from build123d import *

# Parameters (mm, degrees)
F0_W     = 12.7
F0_H     = 5.08
F1_DEPTH = 7.62
F2_R     = 2.53999


# Not quite as in the source:
# - a fillet or chamfer is up to 0.001 mm smaller than in the source, because OpenCascade refuses the exact size


with BuildPart() as f1:
    # F0 (on Top) → F1 (new body)
    with BuildSketch(Plane.XY):
        Polygon((-30.1547096223, 19.9307221919), (-30.1547096223, 5.9384261601), (-19.9947096223, 5.9384261601), (-19.9947096223, 14.8507221919), (-19.9947096223, 19.9307221919), align=None)
        Polygon((-19.9947096223, 5.9384261601), (-30.1547096223, 5.9384261601), (-30.1547096223, -6.7615738399), (33.3452903777, -6.7615738399), (33.3452903777, 5.9384261601), (23.1852903777, 5.9384261601), align=None)
        Polygon((23.1852903777, 14.8507221919), (23.1852903777, 5.9384261601), (33.3452903777, 5.9384261601), (33.3452903777, 19.9307221919), (23.1852903777, 19.9307221919), align=None)
        with Locations((-13.6447096223, 17.3907221919)):
            Rectangle(F0_W, F0_H)
        with Locations((16.8352903777, 17.3907221919)):
            Rectangle(F0_W, F0_H)
    extrude(amount=F1_DEPTH)

    # F2 (radius 2.54 in the source; OpenCascade refuses exactly that, so slightly less here)
    f2_edges = [f1.edges().sort_by_distance(p)[0] for p in [
        (1.59529, -6.761574, 7.62),
        (1.59529, 5.938426, 7.62),
        (-30.15471, 6.584574, 7.62),
        (33.34529, 6.584574, 7.62),
        (21.91529, 19.930722, 7.62),
        (-18.72471, 19.930722, 7.62),
        (21.91529, 19.930722, 0),
        (23.18529, 10.394574, 7.62),
        (16.83529, 14.850722, 7.62),
        (-13.64471, 14.850722, 7.62),
        (1.59529, -6.761574, 0),
        (-30.15471, 6.584574, 0),
        (33.34529, 6.584574, 0),
        (10.48529, 14.850722, 3.81),
        (10.48529, 19.930722, 3.81),
        (-7.29471, 14.850722, 3.81),
        (-7.29471, 19.930722, 3.81),
        (-19.99471, 10.394574, 7.62),
        (1.59529, 5.938426, 0),
        (-19.99471, 10.394574, 0),
        (16.83529, 14.850722, 0),
        (23.18529, 10.394574, 0),
        (-13.64471, 14.850722, 0),
        (10.48529, 17.390722, 0),
        (-7.29471, 17.390722, 0),
        (-18.72471, 19.930722, 0),
        (10.48529, 17.390722, 7.62),
        (-7.29471, 17.390722, 7.62),
    ]]
    fillet(f2_edges, radius=F2_R)


solid = f1.part
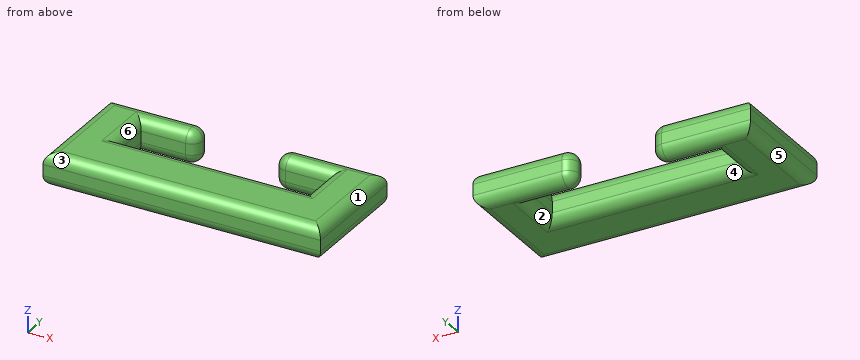
Check sheet for the modelled part. Datum: model origin and axes. Units: mm. Face numbers are marked on the shaded views. A direction names the side the tool comes from. Round coordinates to 2 decimals unless told otherwise and drop trailing zeros. Loops run counter-clockwise (first coordinate to the right, second up) from the corner with the lowest first, then second, coordinate; pieces in that order, holes last.
1. Gauge pin test, flat ends, axial feed: pin 1 Ø5 at (x, y) = (-17, 7.5) entering from -Z; pin 2 Ø3 at (x, y) = (-7, 5) entering from -Z; pin 3 Ø3 at (y, z) = (-4, 2) entering from +X; pin 4 Ø1.3 at (x, z) = (-4.5, 3.5) entering from +Y. Record the tip position at first contact, or that the pin passes through.
2. Scan lines: probe 1 along Y at (x, z) = (19, 3.5); probe 2 along X at (y, z) = (12, 4); probe 3 along X at (y, z) = (6.25, 5.25). Record each from-to range of solid material in increasing order.
3. Mould release check, pull along X, two halves, no side actions. Record for the marked faces 1, 2 and 3: released by +X, released by -X, zero draft, split by the parting line, or undercut.
4. Set-up check for the marked faces 4, 5 and 6: record each of +Z, -Z, +X, -X, +Y, -Y from which the full face is reachable in a straight line by a thin tool's end or side.
5. Sectioned sample at A-A on y = 10.5. Record the boundary of the cut face in (x, z), and give its area (3 significant figures).
6. Sectioned sample at D-D on x = -25. Record the boundary of the cut face in (y, z), and give its area (3 significant figures).
Recorded:
1. pin 1: stops at z = 0.57
1. pin 2: stops at z = 0
1. pin 3: stops at x = 33.35
1. pin 4: stops at y = 5.94
2. probe 1: y = -6.76 to 5.94, 14.85 to 19.93
2. probe 2: x = -30.15 to -19.99, 23.19 to 33.35
2. probe 3: x = -30.15 to -20, 23.19 to 33.34
3. face 1: released by +X
3. face 2: undercut
3. face 3: zero draft
4. face 4: -Z
4. face 5: -Z, -X, +Y, -Y
4. face 6: +Z
5. outline: (-30.15, 2.54) arc R2.54 ccw to (-27.61, 0) - (-22.53, 0) arc R2.54 ccw to (-19.99, 2.54) - (-19.99, 5.08) arc R2.54 ccw to (-22.53, 7.62) - (-27.61, 7.62) arc R2.54 ccw to (-30.15, 5.08) - close; (23.19, 2.54) arc R2.54 ccw to (25.73, 0) - (30.81, 0) arc R2.54 ccw to (33.35, 2.54) - (33.35, 5.08) arc R2.54 ccw to (30.81, 7.62) - (25.73, 7.62) arc R2.54 ccw to (23.19, 5.08) - close
5. area: 144 mm2
6. outline: (-6.76, 2.54) arc R2.54 ccw to (-4.22, 0) - (17.39, 0) arc R2.54 ccw to (19.93, 2.54) - (19.93, 5.08) arc R2.54 ccw to (17.39, 7.62) - (-4.22, 7.62) arc R2.54 ccw to (-6.76, 5.08) - close
6. area: 198 mm2
